```python
from build123d import *

# Parameters (mm, degrees)
SKETCH1_W           = 109.295835398
SKETCH1_H           = 20
SKETCH1_R           = 1.5
SKETCH1_W_2         = 97.295835398
SKETCH1_H_2         = 12
BOSS_EXTRUDE1_DEPTH = 6
CUT_EXTRUDE1_DEPTH  = 112.272546639
FILLET1_R           = 5


with BuildPart() as part:
    # Sketch1 → Boss-Extrude1 (new body)
    with BuildSketch(Plane(origin=(0, 0, 0), x_dir=(1, 0, 0), z_dir=(0, 1, 0))):
        with Locations((54.647917699, 10)):
            Rectangle(SKETCH1_W, SKETCH1_H)
        with Locations(Location((3, 17, 0), (0, 0, 270))):
            Circle(SKETCH1_R, mode=Mode.SUBTRACT)
        with Locations(Location((3, 3, 0), (0, 0, 90))):
            Circle(SKETCH1_R, mode=Mode.SUBTRACT)
        with Locations(Location((106.295835398, 3, 0), (0, 0, 270))):
            Circle(SKETCH1_R, mode=Mode.SUBTRACT)
        with Locations(Location((106.295835398, 17, 0), (0, 0, 90))):
            Circle(SKETCH1_R, mode=Mode.SUBTRACT)
        with Locations((54.647917699, 10)):
            Rectangle(SKETCH1_W_2, SKETCH1_H_2, mode=Mode.SUBTRACT)
    extrude(amount=BOSS_EXTRUDE1_DEPTH)

    # Sketch2 → Cut-Extrude1 (cut, through all)
    with BuildSketch(Plane(origin=(0, 6, 0), x_dir=(1, 0, 0), z_dir=(0, 1, 0))):
        Polygon((90.295835398, 17), (90.295835398, 16), (103.295835398, 16), (103.295835398, 4), (90.295835398, 4), (90.295835398, 3), (104.295835398, 3), (104.295835398, 17), align=None)
    extrude(amount=-CUT_EXTRUDE1_DEPTH, mode=Mode.SUBTRACT)

    # Fillet1
    # the kernel refuses this fillet: 5 mm, written as the material it adds along each edge
    with BuildSketch(Plane(origin=(104.295835398, 6, -17), x_dir=(0, 0, 1), z_dir=(0, -1, 0)), Plane(origin=(104.295835398, 6, -3), x_dir=(-1, 0, 0), z_dir=(0, -1, 0)), Plane(origin=(6, 0, -16), x_dir=(0, 0, 1), z_dir=(0, 1, 0))) as fillet1_piece_1:
        with BuildLine():
            CenterArc((FILLET1_R, FILLET1_R), FILLET1_R, 180, 90)
            Line((0, FILLET1_R), (-FILLET1_R * 0.02, FILLET1_R))
            Line((-FILLET1_R * 0.02, FILLET1_R), (-FILLET1_R * 0.02, -FILLET1_R * 0.02))
            Line((-FILLET1_R * 0.02, -FILLET1_R * 0.02), (FILLET1_R, -FILLET1_R * 0.02))
            Line((FILLET1_R, -FILLET1_R * 0.02), (FILLET1_R, 0))
        make_face()
    extrude(amount=6)
    with BuildSketch(Plane(origin=(90.295835398, 6, -17), x_dir=(1, 0, 0), z_dir=(0, -1, 0))) as fillet1_piece_2:
        with BuildLine():
            CenterArc((3, 5), FILLET1_R, 233.130102354, 36.869897646)
            Line((0, 1), (-0.06, 0.92))
            ThreePointArc((-0.06, 0.92), (-0.1, 0.5), (-0.1, 0))
            Line((-0.1, 0), (0, -0.1))
            Line((0, -0.1), (3, -0.1))
            Line((3, -0.1), (3, 0))
        make_face()
    extrude(amount=6)
    with BuildSketch(Plane(origin=(90.295835398, 6, -3), x_dir=(0, 0, -1), z_dir=(0, -1, 0))) as fillet1_piece_3:
        with BuildLine():
            CenterArc((5, 3), FILLET1_R, 180, 36.869897646)
            Line((0, 3), (-0.1, 3))
            Line((-0.1, 3), (-0.1, 0))
            Line((-0.1, 0), (0, -0.1))
            ThreePointArc((0, -0.1), (0.5, -0.1), (0.92, -0.06))
            Line((0.92, -0.06), (1, 0))
        make_face()
    extrude(amount=6)
    with BuildSketch(Plane(origin=(6, 0, -4), x_dir=(0, 0, -1), z_dir=(0, 1, 0))) as fillet1_piece_4:
        with BuildLine():
            CenterArc((FILLET1_R, -FILLET1_R), FILLET1_R, 90, 90)
            Line((0, -FILLET1_R), (-FILLET1_R * 0.02, -FILLET1_R))
            Line((-FILLET1_R * 0.02, -FILLET1_R), (-FILLET1_R * 0.02, FILLET1_R * 0.02))
            Line((-FILLET1_R * 0.02, FILLET1_R * 0.02), (FILLET1_R, FILLET1_R * 0.02))
            Line((FILLET1_R, FILLET1_R * 0.02), (FILLET1_R, 0))
        make_face()
    extrude(amount=6)


solid = part.part
```
Here's how the part is built. I have some questions about the finished solid (model axes, mm). A direction names the side the tool comes from. Coordinates: 2 decimals unless noted, no trailing zeros. Write each loop counter-clockwise with the first axis right and the second up, starting at its lowest first coordinate (ties: lowest second). Pieces come first, ordered by that corner, then holes. Notation, with made-up numbers: (83, 39) - (107, 39) arc R30 ccw to (107, 77) - close; hole circle Ø11 at (54, 15.25). An arc over 180 degrees is marked (long way). One line per item, written item: value.
1) Suppose I cut it at A-A on x = 3. Write out the boundary of the cut face in (y, z), and give its area (3 significant figures).
Model answer:
outline: (0, -20) - (6, -20) - (6, -18.5) - (0, -18.5) - close; (0, -15.5) - (6, -15.5) - (6, -4.5) - (0, -4.5) - close; (0, -1.5) - (6, -1.5) - (6, 0) - (0, 0) - close
area: 84.0 mm²
2) Suppose I cut it at D-D on y = 4.05. Write out the boundary of the cut face in (x, z).
Model answer:
outline: (0, -20) - (109.3, -20) - (109.3, 0) - (0, 0) - close; hole circle Ø3 at (3, -17); hole circle Ø3 at (3, -3); hole (6, -11) arc R5 ccw to (11, -16) - (90.3, -16) arc R5 ccw to (93.3, -17) - (99.3, -17) arc R5 ccw to (104.3, -12) - (104.3, -8) arc R5 ccw to (99.3, -3) - (93.3, -3) arc R5 ccw to (90.3, -4) - (11, -4) arc R5 ccw to (6, -9) - close; hole circle Ø3 at (106.3, -17); hole circle Ø3 at (106.3, -3)
3) Suppose I cut it at B-B on x = 52.5. Write out the boundary of the cut face in (y, z).
Model answer:
outline: (0, -20) - (6, -20) - (6, -16) - (0, -16) - close; (0, -4) - (6, -4) - (6, 0) - (0, 0) - close
4) I need wall thicknesses on line 1 along Z through (x, y) = (39, 1.95); line 2 along X through (y, z) = (2.4, -3.5); line 3 along Z through (x, y) = (99, 0.85). Which ranges of each line are inside material? Lowest first, please.
Model answer:
line 1: z = -20 to -16, -4 to 0
line 2: x = 0 to 1.59, 4.41 to 91.12, 101.48 to 104.88, 107.71 to 109.3
line 3: z = -20 to -17, -3 to 0
5) We'd pull the mould along Z, two halves only. Please class faces 3 (the flat face through (54, 3, -20)), 4 (the cylindrical face through (8, 3, -15)), 5 (the flat face through (54, 6, -17)): pulls with the +Z half, pulls with the -Z half, needs draft (parallel to the pull), parting line crosses it, or undercut.
Model answer:
face 3: pulls with the -Z half
face 4: undercut
face 5: needs draft
6) Suppose I cut it at C-C on z = -13. Write out the boundary of the cut face in (x, y).
Model answer:
outline: (0, 0) - (6.42, 0) - (6.42, 6) - (0, 6) - close; (104.19, 0) - (109.3, 0) - (109.3, 6) - (104.19, 6) - close
7) On a 3-axis mill with a long thin cutter (end or side, diameter ignored), from which of +Z, -Z, +X, -X, +Y, -Y can I reach the whole of each face in a straight line? I mean faces 1 (the flat face through (54, 3, 0)), 2 (the flat face through (6, 3, -10)). Say none if no direction works.
Model answer:
face 1: +Z, +X, -X, +Y, -Y
face 2: +Y, -Y
8) I'm going to push a flat-ended pin straight in: P1, Ø1.8, axis at x = 106.3, z = -17, coming from the +Y side. Where does the tip first touch, or does it pass through?
Model answer:
P1: passes through
